from build123d import *

# Parameters (mm, degrees)
BOSS_EXTRUDE1_DEPTH = 30
SKETCH3_R           = 2
CUT_EXTRUDE1_DEPTH  = 4
SKETCH5_W           = 2.5
SKETCH5_H           = 23
SKETCH5_W_2         = 8
CUT_EXTRUDE2_DEPTH  = 32


with BuildPart() as part:
    # Sketch2 → Boss-Extrude1 (new body)
    with BuildSketch(Plane.XY):
        Polygon((0, 0), (-31, 0), (-31, 40), (-28, 40), (-28, 3), (0, 3), align=None)
    extrude(amount=BOSS_EXTRUDE1_DEPTH)

    # Sketch3 → Cut-Extrude1 (cut, through all)
    with BuildSketch(Plane(origin=(0, 3, 0), x_dir=(1, 0, 0), z_dir=(0, 1, 0))):
        with Locations((-7, -22.5)):
            Circle(SKETCH3_R)
        with Locations((-21, -22.5)):
            Circle(SKETCH3_R)
        with Locations((-7, -7.5)):
            Circle(SKETCH3_R)
        with Locations((-21, -7.5)):
            Circle(SKETCH3_R)
    extrude(amount=-CUT_EXTRUDE1_DEPTH, mode=Mode.SUBTRACT)

    # Sketch5 → Cut-Extrude2 (cut, through all)
    with BuildSketch(Plane.ZY.offset(31)):
        with Locations((23.5, 18.5)):
            Rectangle(SKETCH5_W, SKETCH5_H)
        with Locations((15, 18.5)):
            Rectangle(SKETCH5_W_2, SKETCH5_H)
        with Locations((6.5, 18.5)):
            Rectangle(SKETCH5_W, SKETCH5_H)
    extrude(amount=-CUT_EXTRUDE2_DEPTH, mode=Mode.SUBTRACT)


solid = part.part
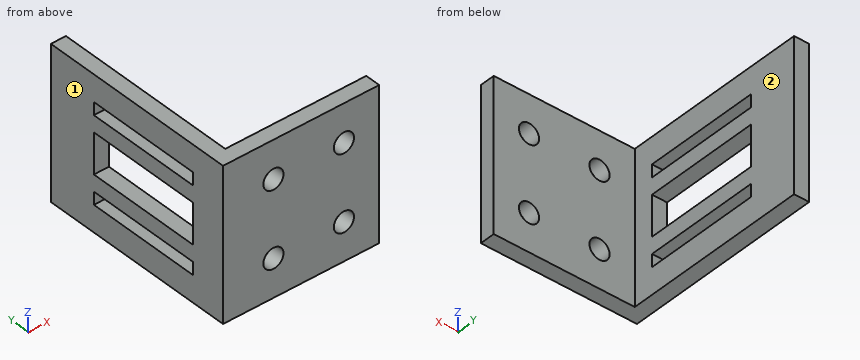
Geometry check sheet. Reference: the model listing, model coordinates, mm. Face numbers are marked on the shaded views. A direction names the side the tool comes from. Round coordinates to 2 decimals unless told otherwise and drop trailing zeros. Order: outer loops, then holes, each group sorted by start corner. A loop starts at its lowest first (then second) coordinate and runs counter-clockwise, first axis right, second up. Notation, with made-up numbers: M 55,75 L 98,75 A17 cw 98,85 Z; hole C 16,86.5 d3. An arc over 180 degrees is marked long. Answer in a Markdown table with one row per item. Add a question column.
Item 1: Sectioned sample at A-A, the plane y = 12. Enter the section's corners in (x, z).
Item 2: Sectioned sample at D-D, the plane z = 27. Enter the section's corners in (x, y).
Item 3: Sectioned sample at C-C, the plane x = -21. Enter the section's corners in (y, z).
Item 4: Material ranges on L1, parallel to Z at x = -7, y = 2.25; L2, parallel to X at y = 0.6, z = 7.5; L3, parallel to Y at x = -15, z = 12.25, recorded low to high. Write a range as [from, to].
Item 5: Sectioned sample at B-B, the plane z = 17.25. Enter the section's corners in (x, y), plus the area to 3 significant figures.
Item 6: Set-up check for the marked faces 1 and 2: record each of +Z, -Z, +X, -X, +Y, -Y from which the full face is reachable in a straight line by a thin tool's end or side.
Item 7: Depth check by flat-ended pin: pin 1 Ø5 at (x, z) = (-17, 3) entering from +Y; pin 2 Ø9 at (y, z) = (24.5, 13) entering from +X. Enter the tip coordinate at first touch or a pass-through.
Filled in:
| question | item | result |
|---|---|---|
| 1 | outline | M -31,0 L -28,0 L -28,5.25 L -31,5.25 Z; M -31,7.75 L -28,7.75 L -28,11 L -31,11 Z; M -31,19 L -28,19 L -28,22.25 L -31,22.25 Z; M -31,24.75 L -28,24.75 L -28,30 L -31,30 Z |
| 2 | outline | M -31,0 L 0,0 L 0,3 L -28,3 L -28,40 L -31,40 Z |
| 3 | outline | M 0,0 L 3,0 L 3,5.5 L 0,5.5 Z; M 0,9.5 L 3,9.5 L 3,20.5 L 0,20.5 Z; M 0,24.5 L 3,24.5 L 3,30 L 0,30 Z |
| 4 | L1 | z = [0, 5.5], [9.5, 20.5], [24.5, 30] |
| 4 | L2 | x = [-31, -23], [-19, -9], [-5, 0] |
| 4 | L3 | y = [0, 3] |
| 5 | outline | M -31,0 L 0,0 L 0,3 L -28,3 L -28,7 L -31,7 Z; M -31,30 L -28,30 L -28,40 L -31,40 Z |
| 5 | area | 135 mm² |
| 6 | face 1 | +Z, -Z, -X, +Y, -Y |
| 6 | face 2 | +Z, -Z, +X, +Y |
| 7 | pin 1 | stops at y = 3 |
| 7 | pin 2 | stops at x = -28 |
